Could you check a few things on this model? Use its own coordinates, in mm. Face numbers are marked on the shaded views. A direction names the side the tool comes from. Give positions to 0.01 mm unless a question says otherwise; leave off trailing zeros. Write each loop counter-clockwise with the first axis right and the second up, starting at its lowest first coordinate (ties: lowest second). Pieces come first, ordered by that corner, then holes. Notation, with made-up numbers: (-22, -35) - (3, -35) arc R4 ccw to (3, -29) - close; hole circle Ø7 at (45, 79.25). An arc over 180 degrees is marked (long way). Answer as CSV lines item,"result". Start each with the question number.
Q1. Imagine slicing it at B-B on y = 3. List the corners of the cut face in (x, z) for me, and give its area (3 significant figures).
Q2. Will these pins go through, and if not, where does the flat tip stop? pin 1 Ø16.5 at (x, z) = (2.5, 10) entering from +Y; pin 2 Ø1.5 at (x, y) = (6.5, 9.5) entering from +Z; pin 3 Ø6 at (x, y) = (-17.5, 12) entering from -Z.
Q3. If I drill on line 1 along X through (y, z) = (11, 0); line 2 along Z through (x, y) = (-10.5, 3.75); line 3 along Z through (x, y) = (1, 3.25), over which ranges is the centre line in solid material (lowest first)?
Q4. On a 3-axis mill with a long thin cutter (end or side, diameter ignored), from which of +Z, -Z, +X, -X, +Y, -Y can I reach the whole of each face in a straight line? I mean the marked faces 4 and 5. Say none if no direction works.
Q5. Imagine slicing it at A-A on z = 0. List the corners of the cut face in (x, y) for me, and give its area (3 significant figures).
Q6. Imagine slicing it at C-C on x = -21.5. List the corners of the cut face in (y, z) for me.
Q7. We'd pull the mould along Z, two halves only. Please class the marked faces 1, 2 and 3: pulls with the +Z half, pulls with the -Z half, needs draft (parallel to the pull), parting line crosses it, or undercut.
Q8. Imagine slicing it at D-D on z = -39. List the corners of the cut face in (x, y) for me, and give its area (3 significant figures).
```python
from build123d import *

# Parameters (mm, degrees)
SKETCH1_W           = 102
SKETCH1_H           = 120
SKETCH1_W_2         = 20
SKETCH1_H_2         = 2
BOSS_EXTRUDE1_DEPTH = 5
CUT_EXTRUDE12_DEPTH = 10
BOSS_EXTRUDE3_START = 10
SKETCH5_R           = 27
SKETCH5_R_2         = 25
BOSS_EXTRUDE3_DEPTH = 10
SKETCH6_W           = 23.5
SKETCH6_H           = 120
CUT_EXTRUDE15_DEPTH = 10


with BuildPart() as part:
    # Sketch1 → Boss-Extrude1 (new body)
    with BuildSketch(Plane(origin=(0, 0, 0), x_dir=(1, 0, 0), z_dir=(0, 1, 0))):
        Rectangle(SKETCH1_W, SKETCH1_H)
        with Locations((0, -11)):
            Rectangle(SKETCH1_W_2, SKETCH1_H_2, mode=Mode.SUBTRACT)
        with Locations((0, 11)):
            Rectangle(SKETCH1_W_2, SKETCH1_H_2, mode=Mode.SUBTRACT)
    extrude(amount=BOSS_EXTRUDE1_DEPTH)

    # Sketch2 → Cut-Extrude12 (cut)
    with BuildSketch(Plane(origin=(0, 5, 0), x_dir=(1, 0, 0), z_dir=(0, 1, 0))):
        with BuildLine():
            Line((3.75, 6.495190528), (12.5, 21.650635095))
            ThreePointArc((12.5, 21.650635095), (0, 25), (-12.5, 21.650635095))
            Line((-12.5, 21.650635095), (-3.75, 6.495190528))
            ThreePointArc((-3.75, 6.495190528), (-7.5, 0), (-3.75, -6.495190528))
            Line((-3.75, -6.495190528), (-12.5, -21.650635095))
            ThreePointArc((-12.5, -21.650635095), (0, -25), (12.5, -21.650635095))
            Line((12.5, -21.650635095), (3.75, -6.495190528))
            ThreePointArc((3.75, -6.495190528), (7.5, 0), (3.75, 6.495190528))
        make_face()
    extrude(amount=-CUT_EXTRUDE12_DEPTH, mode=Mode.SUBTRACT)

    # Sketch5 → Boss-Extrude3 (add)
    with BuildSketch(Plane(origin=(0, 5, 0), x_dir=(1, 0, 0), z_dir=(0, 1, 0)).offset(BOSS_EXTRUDE3_START)):
        with Locations(Location((0, 0, 0), (0, 0, 270))):
            Circle(SKETCH5_R)
        with Locations(Location((0, 0, 0), (0, 0, 270))):
            Circle(SKETCH5_R_2, mode=Mode.SUBTRACT)
    extrude(amount=-BOSS_EXTRUDE3_DEPTH)

    # Sketch6 → Cut-Extrude15 (cut)
    with BuildSketch(Plane(origin=(0, 5, 0), x_dir=(1, 0, 0), z_dir=(0, 1, 0))):
        with Locations((-39.25, 0)):
            Rectangle(SKETCH6_W, SKETCH6_H)
        with Locations((39.25, 0)):
            Rectangle(SKETCH6_W, SKETCH6_H)
    extrude(amount=-CUT_EXTRUDE15_DEPTH, mode=Mode.SUBTRACT)


solid = part.part
```
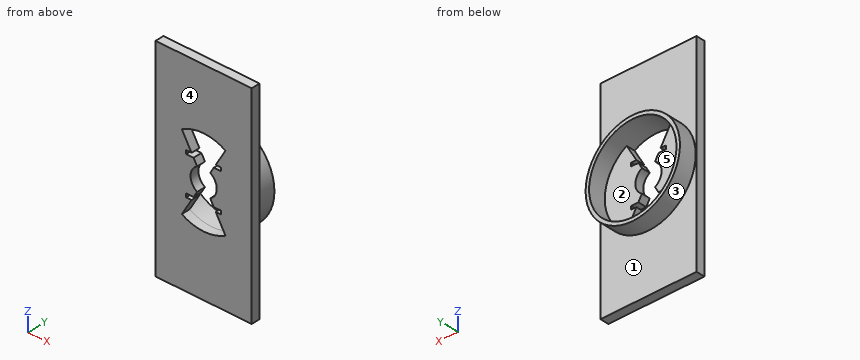
Conclusion:
1,outline,"(-27.5, -60) - (27.5, -60) - (27.5, 60) - (-27.5, 60) - close; hole (-12.5, -21.65) arc R25 ccw to (12.5, -21.65) - (6.93, -12) - (10, -12) - (10, -10) - (5.77, -10) - (3.75, -6.5) arc R7.5 ccw to (3.75, 6.5) - (5.77, 10) - (10, 10) - (10, 12) - (6.93, 12) - (12.5, 21.65) arc R25 ccw to (-12.5, 21.65) - (-6.93, 12) - (-10, 12) - (-10, 10) - (-5.77, 10) - (-3.75, 6.5) arc R7.5 ccw to (-3.75, -6.5) - (-5.77, -10) - (-10, -10) - (-10, -12) - (-6.93, -12) - close"
1,area,"5,800 mm^2"
2,pin 1,"y = 5"
2,pin 2,"z = 26.38"
2,pin 3,"z = -22.78"
3,line 1,"-27 to -25, 25 to 27"
3,line 2,"-60 to -22.69, -18.19 to 18.19, 22.69 to 60"
3,line 3,"-60 to -24.98, 24.98 to 60"
4,face 4,"+Z, -Z, +X, -X, -Y"
4,face 5,"+Y"
5,outline,"(-27.5, 0) - (-7.5, 0) - (-7.5, 5) - (-25, 5) - (-25, 15) - (-27, 15) - (-27, 5) - (-27.5, 5) - close; (7.5, 0) - (27.5, 0) - (27.5, 5) - (27, 5) - (27, 15) - (25, 15) - (25, 5) - (7.5, 5) - close"
5,area,"240 mm^2"
6,outline,"(0, -60) - (5, -60) - (5, -16.33) - (15, -16.33) - (15, -12.76) - (5, -12.76) - (5, 12.76) - (15, 12.76) - (15, 16.33) - (5, 16.33) - (5, 60) - (0, 60) - close"
7,face 1,"needs draft"
7,face 2,"undercut"
7,face 3,"parting line crosses it"
8,outline,"(-27.5, 0) - (27.5, 0) - (27.5, 5) - (-27.5, 5) - close"
8,area,"275 mm^2"
